Build history of the part. All positions in model axes, mm. Face numbers are marked on the shaded views. Coordinates: 2 decimals unless noted, no trailing zeros. Loops run counter-clockwise (first coordinate to the right, second up) from the corner with the lowest first, then second, coordinate; pieces in that order, holes last.
(1) Slice it at B-B (x = -3747). Give the cut face in (y, z), and give its area (3 significant figures).
(2) Flat gauge pins, fed straight in: P1, Ø8, axis at y = -1837.5, z = 25, coming from the -X side; P2, Ø2, axis at y = -1838.5, z = 13.5, coming from the -X side; P3, Ø2, axis at y = -1786.5, z = 53, coming from the +X side. Where does each tip first touch, or does it go through?
(3) Slice it at A-A (z = 62). Give the cut face in (x, y), and give its area (3 significant figures).
(4) Two-plate mould, pull along Z, no slides. Class the marked faces 1 and 2: pulls with the +Z half, pulls with the -Z half, needs draft (parallel to the pull), parting line crosses it, or undercut.
(5) Wall check: L1, parallel to Y at x = -3733, z = -38; L2, parallel to X at y = -1860, z = 67; L3, parallel to Y at x = -3736.5, z = 25.5. Give the ranges that are in metal, low to high.
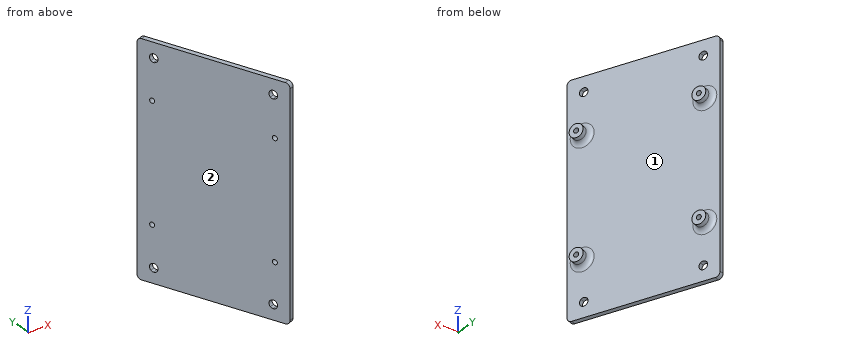
from build123d import *

# Parameters (mm, degrees)
SKETCH1_W           = 152.4
SKETCH1_H           = 97.79
BOSS_EXTRUDE1_DEPTH = 3.175
SKETCH2_R           = 4.445
BOSS_EXTRUDE2_DEPTH = 6.35
FILLET1_R           = 3.175
SKETCH4_R           = 1.6
CUT_EXTRUDE1_DEPTH  = 45.126339074
FILLET2_R           = 3.175
CUT_EXTRUDE2_DEPTH  = 38.776339074


with BuildPart() as part:
    # Sketch1 → Boss-Extrude1 (new body)
    with BuildSketch(Plane(origin=(-3845.744053595, -1594.742620069, 0), x_dir=(0, 0, -1), z_dir=(0.923728021, 0.383049008, 0))):
        with Locations((-2.512437172, -244.506793415)):
            Rectangle(SKETCH1_W, SKETCH1_H)
    extrude(amount=BOSS_EXTRUDE1_DEPTH)

    # Sketch2 → Boss-Extrude2 (add)
    with BuildSketch(Plane(origin=(-3842.811217127, -1593.526439469, 0), x_dir=(0, 0, -1), z_dir=(0.923728021, 0.383049008, 0))):
        with Locations((36.752562828, -283.626793415)):
            Circle(SKETCH2_R)
        with Locations((-41.577437172, -283.626793415)):
            Circle(SKETCH2_R)
        with Locations((-41.577437172, -205.386793415)):
            Circle(SKETCH2_R)
        with Locations((36.752562828, -205.386793415)):
            Circle(SKETCH2_R)
    extrude(amount=BOSS_EXTRUDE2_DEPTH)

    # Fillet1
    fillet1_edges = [part.edges().sort_by_distance(p)[0] for p in [
        (-3734.168255249, -1855.520456151, -32.307562828),
        (-3734.168255249, -1855.520456151, 46.022437172),
        (-3764.13800964, -1783.247975761, 46.022437172),
        (-3764.13800964, -1783.247975761, -32.307562828),
    ]]
    fillet(fillet1_edges, radius=FILLET1_R)

    # Sketch4 → Cut-Extrude1 (cut, through all)
    with BuildSketch(Plane(origin=(-3836.945544191, -1591.094078268, 0), x_dir=(0, 0, -1), z_dir=(0.923728021, 0.383049008, 0))):
        with Locations((36.752562828, -205.386793415)):
            Circle(SKETCH4_R)
        with Locations((-41.577437172, -205.386793415)):
            Circle(SKETCH4_R)
        with Locations((-41.577437172, -283.626793415)):
            Circle(SKETCH4_R)
        with Locations((36.752562828, -283.626793415)):
            Circle(SKETCH4_R)
    extrude(amount=-CUT_EXTRUDE1_DEPTH, mode=Mode.SUBTRACT)

    # Fillet2
    fillet2_edges = [part.edges().sort_by_distance(p)[0] for p in [
        (-3731.890369429, -1865.15798786, -73.687562828),
        (-3731.890369429, -1865.15798786, 78.712437172),
        (-3769.348731928, -1774.826624652, 78.712437172),
        (-3769.348731928, -1774.826624652, -73.687562828),
    ]]
    fillet(fillet2_edges, radius=FILLET2_R)

    # Sketch5 → Cut-Extrude2 (cut, through all)
    with BuildSketch(Plane(origin=(-3842.811217127, -1593.526439469, 0), x_dir=(0, 0, -1), z_dir=(0.923728021, 0.383049008, 0))):
        with BuildLine():
            ThreePointArc((65.787562828, -280.831265324), (63.687562828, -279.856793415), (61.587562828, -280.831265324))
            Line((61.587562828, -280.831265324), (61.587562828, -284.382321505))
            ThreePointArc((61.587562828, -284.382321505), (63.687562828, -285.356793415), (65.787562828, -284.382321505))
            Line((65.787562828, -284.382321505), (65.787562828, -280.831265324))
        make_face()
        with BuildLine():
            Line((61.587562828, -284.382321505), (61.587562828, -280.831265324))
            ThreePointArc((61.587562828, -280.831265324), (60.937562828, -282.606793415), (61.587562828, -284.382321505))
        make_face()
        with BuildLine():
            ThreePointArc((66.437562828, -282.606793415), (66.269955129, -281.661409895), (65.787562828, -280.831265324))
            Line((65.787562828, -280.831265324), (65.787562828, -284.382321505))
            ThreePointArc((65.787562828, -284.382321505), (66.269955129, -283.552176935), (66.437562828, -282.606793415))
        make_face()
        with BuildLine():
            ThreePointArc((65.787562828, -204.631265324), (63.687562828, -203.656793415), (61.587562828, -204.631265324))
            Line((61.587562828, -204.631265324), (61.587562828, -208.182321505))
            ThreePointArc((61.587562828, -208.182321505), (63.687562828, -209.156793415), (65.787562828, -208.182321505))
            Line((65.787562828, -208.182321505), (65.787562828, -204.631265324))
        make_face()
        with BuildLine():
            Line((61.587562828, -208.182321505), (61.587562828, -204.631265324))
            ThreePointArc((61.587562828, -204.631265324), (60.937562828, -206.406793415), (61.587562828, -208.182321505))
        make_face()
        with BuildLine():
            ThreePointArc((66.437562828, -206.406793415), (66.269955129, -205.461409895), (65.787562828, -204.631265324))
            Line((65.787562828, -204.631265324), (65.787562828, -208.182321505))
            ThreePointArc((65.787562828, -208.182321505), (66.269955129, -207.352176935), (66.437562828, -206.406793415))
        make_face()
        with BuildLine():
            Line((-70.812437172, -208.182321505), (-70.812437172, -204.631265324))
            ThreePointArc((-70.812437172, -204.631265324), (-71.462437172, -206.406793415), (-70.812437172, -208.182321505))
        make_face()
        with BuildLine():
            ThreePointArc((-66.612437172, -204.631265324), (-68.712437172, -203.656793415), (-70.812437172, -204.631265324))
            Line((-70.812437172, -204.631265324), (-70.812437172, -208.182321505))
            ThreePointArc((-70.812437172, -208.182321505), (-68.712437172, -209.156793415), (-66.612437172, -208.182321505))
            Line((-66.612437172, -208.182321505), (-66.612437172, -204.631265324))
        make_face()
        with BuildLine():
            ThreePointArc((-65.962437172, -206.406793415), (-66.130044871, -205.461409895), (-66.612437172, -204.631265324))
            Line((-66.612437172, -204.631265324), (-66.612437172, -208.182321505))
            ThreePointArc((-66.612437172, -208.182321505), (-66.130044871, -207.352176935), (-65.962437172, -206.406793415))
        make_face()
        with BuildLine():
            ThreePointArc((-66.612437172, -280.831265324), (-68.712437172, -279.856793415), (-70.812437172, -280.831265324))
            Line((-70.812437172, -280.831265324), (-70.812437172, -284.382321505))
            ThreePointArc((-70.812437172, -284.382321505), (-68.712437172, -285.356793415), (-66.612437172, -284.382321505))
            Line((-66.612437172, -284.382321505), (-66.612437172, -280.831265324))
        make_face()
        with BuildLine():
            ThreePointArc((-65.962437172, -282.606793415), (-66.130044871, -281.661409895), (-66.612437172, -280.831265324))
            Line((-66.612437172, -280.831265324), (-66.612437172, -284.382321505))
            ThreePointArc((-66.612437172, -284.382321505), (-66.130044871, -283.552176935), (-65.962437172, -282.606793415))
        make_face()
        with BuildLine():
            Line((-70.812437172, -284.382321505), (-70.812437172, -280.831265324))
            ThreePointArc((-70.812437172, -280.831265324), (-71.462437172, -282.606793415), (-70.812437172, -284.382321505))
        make_face()
    extrude(amount=-CUT_EXTRUDE2_DEPTH, mode=Mode.SUBTRACT)


solid = part.part
Response values:
1. outline: (-1832.87, -73.69) - (-1824.58, -73.69) - (-1824.58, 78.71) - (-1832.87, 78.71) - close
1. area: 1,260 mm2
2. P1: stops at x = -3746.74
2. P2: stops at x = -3745.08
2. P3: stops at x = -3762.37
3. outline: (-3770.82, -1775.43) - (-3733.36, -1865.77) - (-3730.42, -1864.55) - (-3767.88, -1774.22) - close
3. area: 310 mm2
4. face 1: undercut
4. face 2: needs draft
5. L1: y = -1865.62 to -1856.12, -1853.95 to -1850.41
5. L2: x = -3735.75 to -3732.31
5. L3: y = -1858.19 to -1849.9
